Read the model definition and answer for the solid it produces. Units are mm, in the model's axes. Face numbers are marked on the shaded views. A direction names the side the tool comes from. Coordinates: 2 decimals unless noted, no trailing zeros. Loops run counter-clockwise (first coordinate to the right, second up) from the corner with the lowest first, then second, coordinate; pieces in that order, holes last. Notation, with made-up numbers: (-38, 63) - (-29, 63) arc R18 cw to (-29, 67) - close; hole circle Ø1 at (70, -16.75). An arc over 180 degrees is marked (long way). Use one line per item in the form item = value. Start each with the question number.
1) Which of the six approach directions +Z, -Z, +X, -X, +Y, -Y give full straight-line access (tool end or side, diameter ignored) to the marked faces 1 and 2?
2) A cutting plane is placed at B-B (z = 2.5). Give the vertices of the cut face in (x, y), and give its area (3 significant figures).
3) A cutting plane is placed at D-D (y = 1.9). Give the vertices of the cut face in (x, z), and give its area (3 significant figures).
4) Each of these flat-tipped pins is pushed along its axis until it touches: P1, Ø1, axis at x = 13.5, y = -1.5, coming from the +Z side; P2, Ø1, axis at x = -14.5, y = 0.5, coming from the -Z side; P3, Ø1.5, axis at x = 7.5, y = -0.5, coming from the -Z side. Where does it stop, or does it pass through?
5) The mould has two halves that part along X. Classify the marked faces 3, 4 and 5: released by +X, released by -X, zero draft, split by the parting line, or undercut.
6) A cutting plane is placed at A-A (y = -0.55). Give the vertices of the cut face in (x, z), and give its area (3 significant figures).
7) A cutting plane is placed at C-C (x = 6.5). Give the vertices of the cut face in (y, z), and give its area (3 significant figures).
8) Consider line 1 (X direction, y = -0.1, z = 1.1); line 2 (Y direction, x = 14, z = 0.9); line 3 (Y direction, x = 13, z = 3.2). Determine where each line is inside the solid, lowest interval first.
from build123d import *

# Parameters (mm, degrees)
F0_W     = 42.8
F0_H     = 4.6
F0_W_2   = 40.4
F0_H_2   = 2.2
F1_DEPTH = 3
F2_W     = 42.8
F2_H     = 4.6
F3_DEPTH = 1.5
F5_DEPTH = 40.4
F6_SIZE  = 0.2
F7_R     = 1
F9_DEPTH = 4.1197958302


with BuildPart() as f1:
    # F0 (on Top) → F1 (new body)
    with BuildSketch(Plane.XY):
        Rectangle(F0_W, F0_H)
        Rectangle(F0_W_2, F0_H_2, mode=Mode.SUBTRACT)
    extrude(amount=F1_DEPTH)

    # F2 (on face) → F3 (join)
    with BuildSketch(Plane.XY.offset(3)):
        Rectangle(F2_W, F2_H)
    extrude(amount=F3_DEPTH)

    # F4 (on face) → F5 (cut, through all)
    with BuildSketch(Plane.YZ.offset(-20.2)):
        Polygon((-1.1, 3), (1.1, 3), (0, 4.1), align=None)
    extrude(amount=F5_DEPTH, mode=Mode.SUBTRACT)

    # F6
    f6_edges = [f1.edges().sort_by_distance(p)[0] for p in [
        (0, 1.1, 0),
        (-20.2, 0, 0),
        (0, -1.1, 0),
        (20.2, 0, 0),
    ]]
    chamfer(f6_edges, length=F6_SIZE)

    # F7
    f7_edges = [f1.edges().sort_by_distance(p)[0] for p in [
        (-21.4, -2.3, 2.25),
        (-21.4, 2.3, 2.25),
        (-21.4, 0, 4.5),
        (0, 2.3, 4.5),
        (0, -2.3, 4.5),
        (21.4, -2.3, 2.25),
        (21.4, 0, 4.5),
        (21.4, 2.3, 2.25),
    ]]
    fillet(f7_edges, radius=F7_R)

    # F8 (on face) → F9 (join, up to face)
    with BuildSketch(Plane(origin=(0, 0, 0), x_dir=(1, 0, 0), z_dir=(0, 0, -1))):
        with BuildLine():
            Line((-0.4768552317, -1.3), (0.4768552317, -1.3))
            ThreePointArc((0.4768552317, -1.3), (0, -0.9802041698), (-0.4768552317, -1.3))
        make_face()
    extrude(amount=-F9_DEPTH)


solid = f1.part
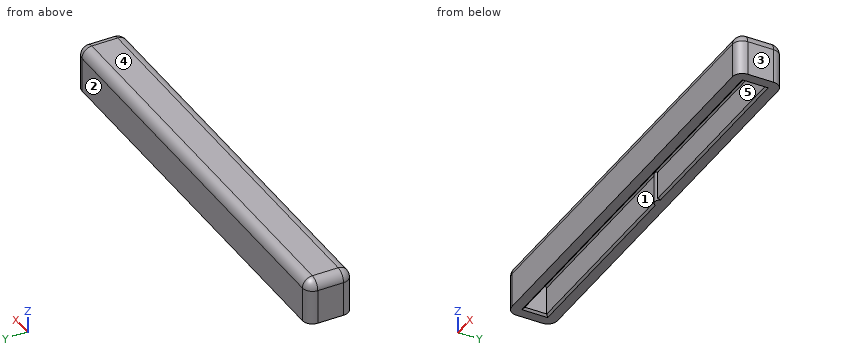
Found:
q1.face_1 = -Z
q1.face_2 = +Z, -Z, +X, -X, +Y
q2.outline = (-21.4, -1.3) arc R1 ccw to (-20.4, -2.3) - (20.4, -2.3) arc R1 ccw to (21.4, -1.3) - (21.4, 1.3) arc R1 ccw to (20.4, 2.3) - (-20.4, 2.3) arc R1 ccw to (-21.4, 1.3) - close; hole (-20.2, -1.1) - (20.2, -1.1) - (20.2, 1.1) - (0.33, 1.1) arc R0.52 cw to (-0.33, 1.1) - (-20.2, 1.1) - close
q2.area = 107 mm^2
q3.outline = (-21.2, 0) - (21.2, 0) - (21.2, 3.5) arc R0.8 ccw to (20.4, 4.3) - (-20.4, 4.3) arc R0.8 ccw to (-21.2, 3.5) - close
q3.area = 182 mm^2
q4.P1 = 4.5
q4.P2 = 3.1
q4.P3 = 0.05
q5.face_3 = released by +X
q5.face_4 = zero draft
q5.face_5 = undercut
q6.outline = (-21.4, 0) - (-20.4, 0) - (-20.2, 0.2) - (-20.2, 3.55) - (20.2, 3.55) - (20.2, 0.2) - (20.4, 0) - (21.4, 0) - (21.4, 3.5) arc R1 ccw to (20.4, 4.5) - (-20.4, 4.5) arc R1 ccw to (-21.4, 3.5) - close
q6.area = 48.7 mm^2
q7.outline = (-2.3, 0) - (-1.3, 0) - (-1.1, 0.2) - (-1.1, 3) - (0, 4.1) - (1.1, 3) - (1.1, 0.2) - (1.3, 0) - (2.3, 0) - (2.3, 3.5) arc R1 ccw to (1.3, 4.5) - (-1.3, 4.5) arc R1 ccw to (-2.3, 3.5) - close
q7.area = 12.4 mm^2
q8.line_1 = -21.4 to -20.2, 20.2 to 21.4
q8.line_2 = -2.3 to -1.1, 1.1 to 2.3
q8.line_3 = -2.3 to -0.9, 0.9 to 2.3
